Design review of the part shown in the three views and the two pictorial views. Dimensions are in mm from the part's minimum x, y and z. A direction names the side the tool comes from. Coordinates: 2 decimals unless noted, no trailing zeros. Write each loop counter-clockwise with the first axis right and the second up, starting at its lowest first coordinate (ties: lowest second). Pieces come first, ordered by that corner, then holes. Notation, with made-up numbers: (-17, -0.5) - (38, -0.5) arc R12 cw to (38, 6.5) - close; hole circle Ø2 at (81.5, -8). An arc over 180 degrees is marked (long way). Write each question's results on one line, items separated by ' | '.
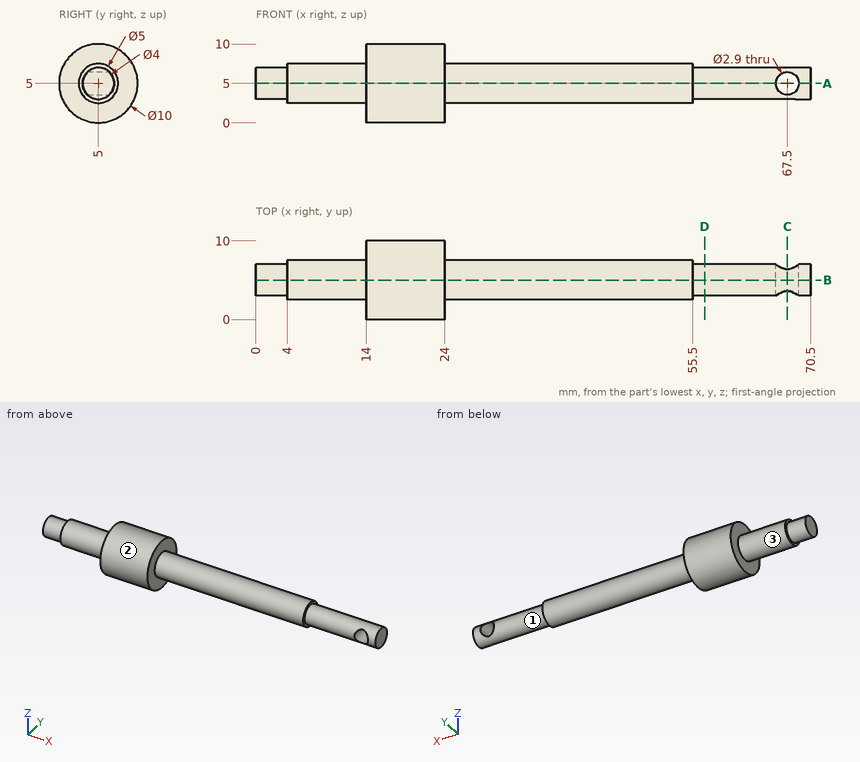
Q1. Take a section at B-B on y = 5. State the section outline as (x, z) points, plus the area to 3 significant figures.
Results found:
outline: (0, 3) - (4, 3) - (4, 2.5) - (14, 2.5) - (14, 0) - (24, 0) - (24, 2.5) - (55.5, 2.5) - (55.5, 3) - (70.5, 3) - (70.5, 7) - (55.5, 7) - (55.5, 7.5) - (24, 7.5) - (24, 10) - (14, 10) - (14, 7.5) - (4, 7.5) - (4, 7) - (0, 7) - close; hole circle Ø2.9 at (67.5, 5) | area: 377 mm2
Q2. Take a section at A-A on z = 5. State the section outline as (x, y) points.
Results found:
outline: (0, 3) - (4, 3) - (4, 2.5) - (14, 2.5) - (14, 0) - (24, 0) - (24, 2.5) - (55.5, 2.5) - (55.5, 3) - (66.05, 3) - (66.05, 7) - (55.5, 7) - (55.5, 7.5) - (24, 7.5) - (24, 10) - (14, 10) - (14, 7.5) - (4, 7.5) - (4, 7) - (0, 7) - close; (68.95, 3) - (70.5, 3) - (70.5, 7) - (68.95, 7) - close
Q3. For pin 1 (2 mm diameter, centred on y = 6.5, z = 1.5, fed in from -X); pin 2 (1.7 mm diameter, centred on x = 67.5, z = 5, fed in from +Y); pin 3 (3 mm diameter, centred on x = 11, y = 2, fed in from -Z); pin 4 (1 mm diameter, centred on y = 3, z = 2.5, fed in from +X), all flat-tipped, find the tip position at first contact; note any pin that passes through.
Results found:
pin 1: x = 14 | pin 2: through | pin 3: z = 3 | pin 4: x = 24
Q4. Take a section at C-C on x = 67.5. State the section outline as (y, z) points, plus the area to 3 significant figures.
Results found:
outline: (3.62, 3.55) arc R2 ccw to (6.38, 3.55) - close; (3.62, 6.45) - (6.38, 6.45) arc R2 ccw to start | area: 2.08 mm2
Q5. For the marked faces 1, 2 and 3, list the 3-axis set-ups (+Z, -Z, +X, -X, +Y, -Y) from which the entire face can be reached by the end or side of a thin tool; tool diameter is ignored.
Results found:
face 1: +X | face 2: +X, -X | face 3: -X
Q6. Take a section at D-D on x = 57. State the section outline as (y, z) points, plus the area to 3 significant figures.
Results found:
outline: circle Ø4 at (5, 5) | area: 12.6 mm2
Q7. Wall thickness on line 1 along X through (y, z) = (5.5, 5); line 2 along Z through (x, y) = (26, 5); line 3 along X through (y, z) = (4.5, 9): over which ranges is each line inside the solid? List them lowest first. Write a range as from..to.
Results found:
line 1: 0..66.05, 68.95..70.5 | line 2: 2.5..7.5 | line 3: 14..24
